from build123d import *

# Parameters (mm, degrees)
F0_W     = 56.2
F0_H     = 38
F1_DEPTH = 23.2
F2_R     = 5
F3_R     = 10
F4_DEPTH = 13


with BuildPart() as f1:
    # F0 (on Top) → F1 (new body)
    with BuildSketch(Plane.XY):
        Rectangle(F0_W, F0_H)
    extrude(amount=F1_DEPTH)

    # F2
    f2_edges = [f1.edges().sort_by_distance(p)[0] for p in [
        (28.1, -19, 11.6),
        (28.1, 19, 11.6),
        (-28.1, 19, 11.6),
        (-28.1, -19, 11.6),
    ]]
    fillet(f2_edges, radius=F2_R)

    # F3 (on face) → F4 (join)
    with BuildSketch(Plane.YZ.offset(28.1)):
        with Locations((0, 11.6)):
            Circle(F3_R)
    extrude(amount=F4_DEPTH)


solid = f1.part
Part model, mm, in its own coordinate system. A direction names the side the tool comes from. Round coordinates to 2 decimals unless told otherwise and drop trailing zeros. Write each loop counter-clockwise with the first axis right and the second up, starting at its lowest first coordinate (ties: lowest second). Pieces come first, ordered by that corner, then holes. Notation, with made-up numbers: (54.25, -12.5) - (92.25, -12.5) arc R32 ccw to (92.25, 16.5) - close; hole circle Ø3 at (32.5, 43.25). An arc over 180 degrees is marked (long way). Use CSV: the item, a comma, the result in double quotes.
Item 1: Flat gauge pins, fed straight in: P1, Ø1, axis at x = 27.5, z = 3, coming from the -Y side; P2, Ø1, axis at x = 26, z = 16.5, coming from the -Y side; P3, Ø1, axis at y = -12, z = 14.5, coming from the +X side. Where does each tip first touch, or does it go through?
Results list:
P1,"stops at y = -17.13"
P2,"stops at y = -18.39"
P3,"stops at x = 28.1"
Item 2: Wall check: L1, parallel to X at y = -11, z = 5.25; L2, parallel to Y at x = 30.5, z = 5; L3, parallel to Y at x = 36, z = 6. Give the ranges that are in metal, low to high.
Results list:
L1,"x = -28.1 to 28.1"
L2,"y = -7.51 to 7.51"
L3,"y = -8.28 to 8.28"
Item 3: Slice it at A-A, the plane y = 0. Write the cut outline in (x, z).
Results list:
outline,"(-28.1, 0) - (28.1, 0) - (28.1, 1.6) - (41.1, 1.6) - (41.1, 21.6) - (28.1, 21.6) - (28.1, 23.2) - (-28.1, 23.2) - close"
Item 4: Slice it at D-D, the plane z = 5. Write the cut outline in (x, y).
Results list:
outline,"(-28.1, -14) arc R5 ccw to (-23.1, -19) - (23.1, -19) arc R5 ccw to (28.1, -14) - (28.1, -7.51) - (41.1, -7.51) - (41.1, 7.51) - (28.1, 7.51) - (28.1, 14) arc R5 ccw to (23.1, 19) - (-23.1, 19) arc R5 ccw to (-28.1, 14) - close"
Item 5: Slice it at B-B, the plane z = 11.6. Write the cut outline in (x, y).
Results list:
outline,"(-28.1, -14) arc R5 ccw to (-23.1, -19) - (23.1, -19) arc R5 ccw to (28.1, -14) - (28.1, -10) - (41.1, -10) - (41.1, 10) - (28.1, 10) - (28.1, 14) arc R5 ccw to (23.1, 19) - (-23.1, 19) arc R5 ccw to (-28.1, 14) - close"
Item 6: Tool access for faces 1 (the flat face through (-28.1, 0, 11)), 2 (the cylindrical face through (34.509, -1.302, 21.515)): list every direction of +Z, -Z, +X, -X, +Y, -Y with a clear straight run to the whole face (end or side of a thin tool).
Results list:
face 1,"+Z, -Z, -X, +Y, -Y"
face 2,"+X"
Item 7: Slice it at C-C, the plane y = 6. Write the cut outline in (x, z).
Results list:
outline,"(-28.1, 0) - (28.1, 0) - (28.1, 3.6) - (41.1, 3.6) - (41.1, 19.6) - (28.1, 19.6) - (28.1, 23.2) - (-28.1, 23.2) - close"
